Autodesk Inventor part; units mm, degrees
ref_plane "Work Plane3" through (0, 3.175, 6.35) normal (1, 0, 0) x (0, -1, 0)
ref_plane "Work Plane4" through (0, 2.5647, -7.8406) normal (-1, 0, 0) x (0, 0, 1)
ref_plane "YZ Plane" through (0, 0, 0) normal (1, 0, 0) x (0, 1, 0)
sketch "Sketch1" plane through (0, 0, 0) normal (1, 0, 0) x (0, 1, 0)
  line L0 (-1.3067, 0) -> (7.8401, 0) construction
  line L1 (0, -10.9768) -> (0, 10.9768) construction
  line L2 (0, -1.7272) -> (0, -6.35)
  line L3 (0, -1.7272) -> (0, -1.7272)
  line L4 (0, -1.7272) -> (3.175, -3.5603)
  line L5 (3.175, -3.5603) -> (3.175, -6.35)
  line L6 (3.175, -6.35) -> (0, -6.35)
  circle A0 centre (3.3584, 0) radius 3.175 construction
  line L7 (2.5647, 7.8406) -> (4.1522, 7.8406) construction
  line L8 (4.1522, 7.8406) -> (4.1522, -7.8406) construction
  line L9 (4.1522, -7.8406) -> (2.5647, -7.8406) construction
  line L10 (2.5647, -7.8406) -> (2.5647, 7.8406) construction
  line L11 (2.5647, 7.8406) -> (4.1522, -7.8406) construction
  line L12 (4.1522, 7.8406) -> (2.5647, -7.8406) construction
  line L13 (0, 1.7272) -> (0, 6.35)
  line L14 (0, 1.7272) -> (0, 1.7272)
  line L15 (0, 1.7272) -> (3.175, 3.5603)
  line L16 (3.175, 3.5603) -> (3.175, 6.35)
  line L17 (3.175, 6.35) -> (0, 6.35)
  point P0 (0, 0)
  point P1 (2.3851, -3.0222)
  point P2 (2.3851, 3.0222)
  dimension "d12" = 60
  dimension "d13" = 0
  dimension "bearing_thickness" = 3.175
  dimension "d15" = 1.7272
  dimension "d17" = 6.35
  dimension "d18" = 1.5875
  dimension "d23" = 12.7
  dimension "d52" = 3.3584
sketch "Sketch11" plane through (0, 0, 0) normal (1, 0, 0) x (0, 1, 0)
  line L0 (3.175, 6.35) -> (0, 6.35)
  line L1 (3.175, -6.35) -> (0, -6.35)
  line L2 (-1.3067, 0) -> (7.8401, 0) construction
  line L3 (0, -10.9768) -> (0, 10.9768) construction
  line L4 (3.175, 6.35) -> (3.175, 0.762)
  line L5 (3.175, 0.762) -> (0, 0.762)
  line L6 (0, 6.35) -> (0, 0.762)
  line L7 (3.175, -6.35) -> (0, -6.35)
  line L8 (0, 10.9768) -> (0, -10.9768) construction
  line L9 (3.175, -6.35) -> (3.175, -0.762)
  line L10 (3.175, -0.762) -> (0, -0.762)
  line L11 (0, -6.35) -> (0, -0.762)
  point P0 (0, 0)
  dimension "d54" = 5.588
extrude "Extrusion4" add sketch "Sketch11" along normal blind 3.556 and the other way blind 14.224
sketch "Sketch17" plane through (3.556, 0, 0) normal (1, 0, 0) x (0, 0, -1)
  line L0 (-6.35, 3.175) -> (-0.762, 3.175)
  line L1 (-0.762, 3.175) -> (0.762, 3.175)
  line L2 (0.762, 3.175) -> (0.762, 0)
  line L3 (0.762, 0) -> (-0.762, 0)
  line L4 (-0.762, 0) -> (-0.762, 3.175)
  point P0 (0, 0)
ref_plane "Work Plane3" through (0, 3.175, 6.35) normal (1, 0, 0) x (0, -1, 0)
extrude "Extrusion6" add sketch "Sketch17" against normal blind 17.78
sketch "Sketch14" plane through (-14.224, 3.175, -6.35) normal (0, 1, 0) x (1, 0, 0)
  line L0 (-3.556, -6.35) -> (21.336, -6.35)
  line L1 (0, -5.588) -> (0, 0)
  point P0 (14.224, -6.35)
  point P1 (2.54, -2.794)
  point P2 (7.112, -2.794)
  point P3 (2.54, -9.906)
  point P4 (7.112, -9.906)
  dimension "d65" = 7.112
  dimension "d66" = 11.684
  dimension "d67" = 3.556
hole "Hole2" at (-11.684, 3.175, -3.556) at (-7.112, 3.175, -3.556) at (-11.684, 3.175, 3.556) at (-7.112, 3.175, 3.556) direction (0, -1, 0) diameter 2.4384 depth 6.6294 tip angle 118 countersink diameter 4.3688 countersink angle 82
sketch "Sketch12" plane through (0, 3.175, 6.35) normal (1, 0, 0) x (0, -1, 0)
  line L0 (3.175, 4.6228) -> (0, 2.7897)
  line L1 (3.175, 8.0772) -> (0, 9.9103)
  line L2 (4.4817, 6.35) -> (-4.6651, 6.35) construction
  line L3 (3.175, 17.3268) -> (3.175, -4.6268) construction
  line L4 (3.175, 4.6228) -> (3.175, 7.0113)
  line L5 (3.175, 4.6228) -> (3.175, 4.6228)
  line L6 (3.175, 8.0772) -> (3.175, 8.0772)
  line L7 (3.175, 7.0113) -> (3.175, 8.0772)
  line L8 (0, 2.7897) -> (0, 9.9103)
  line L9 (0, 0) -> (0, 5.588)
  point P0 (3.175, 6.35)
extrude "Extrusion5" [suppressed]
ref_plane "Work Plane4" through (0, 2.5647, -7.8406) normal (-1, 0, 0) x (0, 0, 1)
sketch "Sketch16" plane through (0, 2.5647, -7.8406) normal (-1, 0, 0) x (0, 0, 1)
  line L0 (6.1134, -2.5647) -> (4.2803, 0.6103)
  line L1 (9.5678, -2.5647) -> (11.4008, 0.6103)
  line L2 (11.4008, 0.6103) -> (4.2803, 0.6103)
  line L3 (7.1793, -2.5647) -> (6.1134, -2.5647)
  line L4 (9.5678, -2.5647) -> (7.1793, -2.5647)
  line L5 (9.5678, -2.5647) -> (9.5678, -2.5647)
  line L6 (6.1134, -2.5647) -> (6.1134, -2.5647)
  line L7 (7.8406, -3.8713) -> (7.8406, 5.2754)
  line L8 (7.8406, 0.6103) -> (7.8406, -2.5647)
revolve "Revolution7" cut sketch "Sketch16" angle 360 about axis through (0, 3.175, 0) along (0, -1, 0) contours L2 L1 L4 L7
sketch "Sketch13" plane through (0, 3.175, 6.35) normal (1, 0, 0) x (0, -1, 0)
  circle A0 centre (-0.1834, 6.35) radius 3.175
  line L0 (4.4817, 6.35) -> (-4.6651, 6.35) construction
  line L1 (-3.3584, 6.35) -> (2.9916, 6.35)
  point P0 (3.175, 6.35)
revolve "Revolution6" cut sketch "Sketch13" angle 360 about axis through (0, 6.5334, 0) along (0, -1, 0)
equation "\"d12\" = bearing_angle"
equation "\"hole1_setback_qq\" = 7.112"
equation "\"hole_lateral_qq\" = 3.556"
equation "\"hole2_setback_qq\" = 11.684"
equation "\"bearing_angle_qq\" = 60deg"
equation "\"bearing_spacing_qq\" = 1.7272"
properties part number "v2_bearing_insert_thick_round" material "Stainless Steel, 440C"
Input: part model. Units: mm. Frame: model coordinates. Give positions to 0.01 mm unless a question says otherwise; leave off trailing zeros. Order: outer loops, then holes, each group sorted by start corner. A loop starts at its lowest first (then second) coordinate and runs counter-clockwise, first axis right, second up.
Q1. Ray query, probe 1 along X at (y, z) = (3.05, 2); probe 2 along Z at (x, y) = (-7.75, 1); probe 3 along X at (y, z) = (0.45, 2.5). Return the intervals inside material, ascending.
Checked values:
probe 1: x = -14.22 to -13.06, -10.31 to -8.49, -5.74 to -2.86, 2.86 to 3.56
probe 2: z = -6.35 to -4.59, -2.52 to 2.52, 4.59 to 6.35
probe 3: x = -14.22 to -12.29, -11.07 to -7.72, -6.5 to 3.56
Q2. Contact query for flat-ended pins moving along their axis: pin 1 Ø3 at (x, z) = (-7.112, 3.556) entering from +Y; pin 2 Ø2 at (x, z) = (-7.5, 3) entering from +Y; pin 3 Ø3 at (x, z) = (1.5, -2) entering from +Y (3 decimals). Output: stop coordinate, or through.
Checked values:
pin 1: stops at y = 2.39
pin 2: stops at y = 2.59
pin 3: stops at y = 3.175
Q3. Draft query along X for faces 1 (the flat face through (3.556, 2, 0)), 2 (the cylindrical face through (-5.922, 1.018, 3.292)), 3 (the flat face through (-5, 2, -6.35)). Return one class per face: +X half, -X half, draft (parallel to the pull), parting line (faces both ways), or undercut.
Checked values:
face 1: +X half
face 2: undercut
face 3: draft
Q4. Section B-B on y = 2.8. Output: boundary loops of the cut face in (x, z), and give its area (3 significant figures).
Checked values:
outline: (-14.22, -6.35) - (3.56, -6.35) - (3.56, 6.35) - (-14.22, 6.35) - close; hole circle Ø3.72 at (-11.68, -3.56); hole circle Ø3.72 at (-11.68, 3.56); hole circle Ø3.72 at (-7.11, -3.56); hole circle Ø3.72 at (-7.11, 3.56); hole circle Ø6.69 at (0, 0)
area: 147 mm2
Q5. Section C-C on x = -12. State how many separate pieces and enclosed holes the cut face has, and give its area (3 significant figures).
Checked values:
separate pieces: 3
enclosed holes: 0
area: 23.2 mm2
Q6. Section A-A on x = 0. Output: boundary loops of the cut face in (y, z) (3 decimals).
Checked values:
outline: (0, -6.35) - (3.175, -6.35) - (3.175, -3.56) - (1.785, -2.758) arc R3.175 cw to (1.757, -2.741) - (0, -1.727) - close; (0, 1.727) - (1.757, 2.741) arc R3.175 cw to (1.785, 2.758) - (3.175, 3.56) - (3.175, 6.35) - (0, 6.35) - close
